Model file for the job. Use its own axes, mm. Face numbers are marked on the shaded views. Give positions to 0.01 mm unless a question says otherwise; leave off trailing zeros. Loops run counter-clockwise (first coordinate to the right, second up) from the corner with the lowest first, then second, coordinate; pieces in that order, holes last. Notation, with made-up numbers: (-31, 27.5) - (24, 27.5) arc R31 ccw to (24, 53.5) - close; hole circle Ø1 at (33.5, 50). An arc over 180 degrees is marked (long way). Answer as CSV lines item,"result". Start each with the question number.
Item 1: Drill centre lines: L1, parallel to Y at x = 29.5, z = 0.35; L2, parallel to X at y = -38.5, z = 1.3; L3, parallel to X at y = -41, z = 1.35. Where is each one in solid material? Low to high. Write a range as from..to.
Item 2: Saw through at B-B on x = 15. Give the cut face in (y, z).
Item 3: Saw through at C-C on y = 10. Give the cut face in (x, z).
Item 4: Saw through at A-A on z = 1.7. Give the cut face in (x, y), plus the area to 3 significant figures.
Item 5: Saw through at D-D on x = 30. Give the cut face in (y, z), plus the area to 3 significant figures.
Item 6: Pull direction Y, two halves, no side cores. Call the marked faces 1, 2 and 3: pulls with the +Y half, pulls with the -Y half, needs draft (parallel to the pull), parting line crosses it, or undercut.
Item 7: Pin check, flat tips, straight feed: pin 1 (1 mm diameter, centred on y = -24, z = 1, fed in from +X); pin 2 (3 mm diameter, centred on x = -23.5, z = 4, fed in from +Y); pin 3 (2 mm diameter, centred on x = 3, z = 3.5, fed in from +Y). Stop position of each tip, or through.
from build123d import *

# Parameters (mm, degrees)
SKETCH_1_R          = 49
SKETCH_1_R_2        = 3.3
EXTRUDE_1_DEPTH     = 6
SKETCH_2_R          = 5
CUT_EXTRUDE_1_DEPTH = 70.555733049


with BuildPart() as part:
    # 草图1 → 凸台-拉伸1 (new body)
    with BuildSketch(Plane.XY.offset(6)):
        with Locations(Location((0, 0, 0), (0, 0, 180))):
            Circle(SKETCH_1_R)
        with Locations(Location((15, 40.300002161, 0), (0, 0, 180))):
            Circle(SKETCH_1_R_2, mode=Mode.SUBTRACT)
        with Locations(Location((15, -40.300002161, 0), (0, 0, 180))):
            Circle(SKETCH_1_R_2, mode=Mode.SUBTRACT)
        with Locations(Location((-15, 40.300002161, 0), (0, 0, 180))):
            Circle(SKETCH_1_R_2, mode=Mode.SUBTRACT)
        with Locations(Location((-15, -40.300002161, 0), (0, 0, 180))):
            Circle(SKETCH_1_R_2, mode=Mode.SUBTRACT)
    extrude(amount=-EXTRUDE_1_DEPTH)

    # 草图2 → 切除-拉伸1 (cut, through all)
    with BuildSketch(Plane.XY.offset(6)):
        with Locations((30, 10)):
            Circle(SKETCH_2_R)
        with Locations((30, -10)):
            Circle(SKETCH_2_R)
    extrude(amount=-CUT_EXTRUDE_1_DEPTH, mode=Mode.SUBTRACT)


solid = part.part
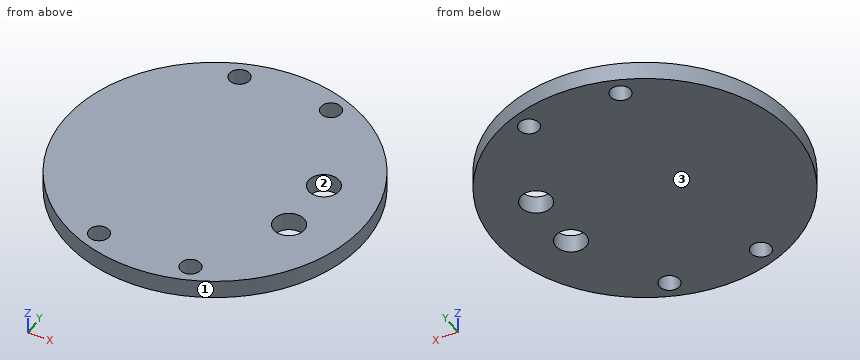
Responses:
1,L1,"-39.12..-14.97, -5.03..5.03, 14.97..39.12"
1,L2,"-30.31..-17.77, -12.23..12.23, 17.77..30.31"
1,L3,"-26.83..-18.22, -11.78..11.78, 18.22..26.83"
2,outline,"(-46.65, 0) - (-43.6, 0) - (-43.6, 6) - (-46.65, 6) - close; (-37, 0) - (37, 0) - (37, 6) - (-37, 6) - close; (43.6, 0) - (46.65, 0) - (46.65, 6) - (43.6, 6) - close"
3,outline,"(-47.97, 0) - (25, 0) - (25, 6) - (-47.97, 6) - close; (35, 0) - (47.97, 0) - (47.97, 6) - (35, 6) - close"
4,outline,"circle Ø98 at (0, 0); hole circle Ø6.6 at (-15, -40.3); hole circle Ø6.6 at (-15, 40.3); hole circle Ø6.6 at (15, -40.3); hole circle Ø6.6 at (15, 40.3); hole circle Ø10 at (30, -10); hole circle Ø10 at (30, 10)"
4,area,"7,250 mm2"
5,outline,"(-38.74, 0) - (-15, 0) - (-15, 6) - (-38.74, 6) - close; (-5, 0) - (5, 0) - (5, 6) - (-5, 6) - close; (15, 0) - (38.74, 0) - (38.74, 6) - (15, 6) - close"
5,area,"345 mm2"
6,face 1,"parting line crosses it"
6,face 2,"undercut"
6,face 3,"needs draft"
7,pin 1,"x = 43"
7,pin 2,"y = 43.78"
7,pin 3,"y = 48.96"
